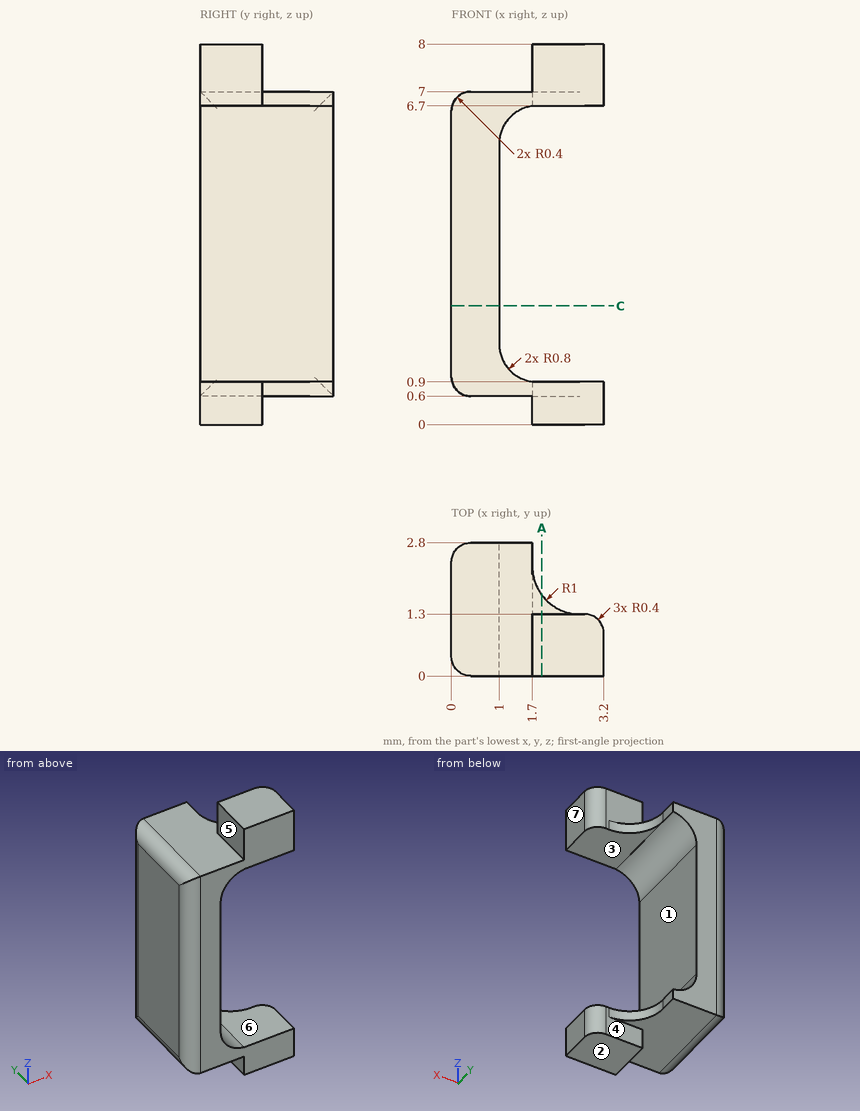
For this review, use the dimensioned drawing (mm, ordinates from the lowest corner) and the shaded views. A direction names the side the tool comes from. Coordinates: 2 decimals unless noted, no trailing zeros. Loops run counter-clockwise (first coordinate to the right, second up) from the corner with the lowest first, then second, coordinate; pieces in that order, holes last. Notation, with made-up numbers: (-36.5, -11.5) -> (15.5, -11.5) arc R26 cw to (15.5, 14.5) -> close; hole circle Ø7 at (-12, -16.75). An arc over 180 degrees is marked (long way). Return JSON: item names as keys, results as strings. Group by question number.
(1) For pin 1 Ø0.7 at (x, y) = (2, 2) entering from +Z; pin 2 Ø0.8 at (y, z) = (0.5, 7.5) entering from -X; pin 3 Ø0.9 at (x, z) = (2.5, 7) entering from +Y, all flat-tipped, find the tip position at first contact; note any pin that passes through.
(2) Consider section A-A, the plane x = 1.9. Give the boundary of the cut face in (y, z), plus the area to 3 significant figures.
(3) Tool access review of the marked faces 5, 6 and 7: name each direction out of +Z, -Z, +X, -X, +Y, -Y from which nothing blocks a thin tool from reaching the whole face with its end or side.
(4) Consider section C-C, the plane z = 2.5. Give the boundary of the cut face in (x, y).
(5) To check wall thickness, follow L1, parallel to Z at x = 2.35, y = 0.55; L2, parallel to Z at x = 0.9, y = 1.65; L3, parallel to X at y = 2.1, z = 3.25. State the ranges of each line that lie inside material, in increasing order.
(6) Mouldability with a two-part tool opening along Z and no side actions: class the marked faces 1, 2, 3 and 4 as pulls with the +Z half, pulls with the -Z half, needs draft (parallel to the pull), parting line crosses it, or undercut.
Results below:
{
 "1": {"pin 1": "stops at z = 7", "pin 2": "stops at x = 1.7", "pin 3": "stops at y = 1.54"},
 "2": {"outline": "(0, 0) -> (1.3, 0) -> (1.3, 0.6) -> (1.7, 0.6) -> (1.7, 0.9) -> (0, 0.9) -> close; (0, 6.7) -> (1.7, 6.7) -> (1.7, 7) -> (1.3, 7) -> (1.3, 8) -> (0, 8) -> close", "area": "3.10 mm2"},
 "3": {"face 5": "+Z, -X, +Y, -Y", "face 6": "+X, +Y, -Y", "face 7": "+Z, -Z, +X, +Y, -Y"},
 "4": {"outline": "(0, 0.4) arc R0.4 ccw to (0.4, 0) -> (1, 0) -> (1, 2.8) -> (0.4, 2.8) arc R0.4 ccw to (0, 2.4) -> close"},
 "5": {"L1": "z = 0 to 0.9, 6.7 to 8", "L2": "z = 0.6 to 7", "L3": "x = 0 to 1"},
 "6": {"face 1": "undercut", "face 2": "pulls with the -Z half", "face 3": "undercut", "face 4": "needs draft"}
}
